For this review, take the finished solid that the model builds, in its own axes (mm). A direction names the side the tool comes from. Round coordinates to 2 decimals unless told otherwise and drop trailing zeros. Order: outer loops, then holes, each group sorted by start corner. A loop starts at its lowest first (then second) coordinate and runs counter-clockwise, first axis right, second up. Notation, with made-up numbers: (10.5, 89.25) -> (60.5, 89.25) arc R17 cw to (60.5, 113.25) -> close; hole circle Ø3 at (18.25, 17.5). An arc over 180 degrees is marked (long way). Answer in a Markdown table with one row per item.
```python
from build123d import *
from build123d.topology import SkipClean

# Parameters (mm, degrees)
SKETCH1_R           = 4
SKETCH1_R_2         = 13
BOSS_EXTRUDE1_DEPTH = 3
BOSS_EXTRUDE2_START = 5
SKETCH2_R           = 17
SKETCH2_R_2         = 8
BOSS_EXTRUDE2_DEPTH = 5
SKETCH3_R           = 1.55
SKETCH3_R_2         = 1
CUT_EXTRUDE1_DEPTH  = 8
SKETCH4_R           = 3.5
SKETCH4_R_2         = 2.2
CUT_EXTRUDE2_DEPTH  = 4.5
SKETCH5_W           = 50
SKETCH5_H           = 15
SKETCH5_R           = 1.55
BOSS_EXTRUDE3_DEPTH = 5
SKETCH9_W           = 42.373333334
SKETCH9_H           = 64.15
BOSS_EXTRUDE6_DEPTH = 3
SKETCH11_R          = 1.55
SKETCH11_R_2        = 4.5
BOSS_EXTRUDE7_DEPTH = 5
SKETCH12_R          = 1.55
BOSS_EXTRUDE8_DEPTH = 4
SKETCH13_R          = 3.5
CUT_EXTRUDE3_DEPTH  = 3


with BuildPart() as part:
    # Sketch1 → Boss-Extrude1 (new body)
    with BuildSketch(Plane.XY):
        with BuildLine():
            Line((-25, 0), (25, 0))
            Line((25, 0), (17, 150))
            ThreePointArc((17, 150), (0, 167), (-17, 150))
            Line((-17, 150), (-25, 0))
        make_face()
        with Locations((0, 150)):
            Circle(SKETCH1_R, mode=Mode.SUBTRACT)
        with Locations((0, 90)):
            Circle(SKETCH1_R_2, mode=Mode.SUBTRACT)
    extrude(amount=BOSS_EXTRUDE1_DEPTH)

    # Sketch2 → Boss-Extrude2 (add)
    with SkipClean():  # the faces are left unmerged after this step: merging them gives an invalid solid
        with BuildSketch(Plane(origin=(0, 0, 0), x_dir=(-1, 0, 0), z_dir=(0, 0, -1)).offset(BOSS_EXTRUDE2_START)):
            with Locations((0, 150)):
                Circle(SKETCH2_R)
            with Locations((0, 150)):
                Circle(SKETCH2_R_2, mode=Mode.SUBTRACT)
        extrude(amount=-BOSS_EXTRUDE2_DEPTH)

    # Sketch3 → Cut-Extrude1 (cut)
    with SkipClean():  # the faces are left unmerged after this step: merging them gives an invalid solid
        with BuildSketch(Plane.XY.offset(3)):
            with Locations((-12.5, 150)):
                Circle(SKETCH3_R)
            with Locations((0, 162.5)):
                Circle(SKETCH3_R)
            with Locations((12.5, 150)):
                Circle(SKETCH3_R)
            with Locations((0, 137.5)):
                Circle(SKETCH3_R)
            with Locations((8.980256121, 158.980256121)):
                Circle(SKETCH3_R_2)
            with Locations((8.980256121, 141.019743879)):
                Circle(SKETCH3_R_2)
            with Locations((-8.980256121, 141.019743879)):
                Circle(SKETCH3_R_2)
            with Locations((-8.980256121, 158.980256121)):
                Circle(SKETCH3_R_2)
        extrude(amount=-CUT_EXTRUDE1_DEPTH, mode=Mode.SUBTRACT)

    # Sketch4 → Cut-Extrude2 (cut)
    with SkipClean():  # the faces are left unmerged after this step: merging them gives an invalid solid
        with BuildSketch(Plane.XY.offset(3)):
            with Locations((-12.5, 150)):
                Circle(SKETCH4_R)
            with Locations((0, 162.5)):
                Circle(SKETCH4_R)
            with Locations((12.5, 150)):
                Circle(SKETCH4_R)
            with Locations((0, 137.5)):
                Circle(SKETCH4_R)
            with Locations((-8.980256121, 158.980256121)):
                Circle(SKETCH4_R_2)
            with Locations((8.980256121, 158.980256121)):
                Circle(SKETCH4_R_2)
            with Locations((8.980256121, 141.019743879)):
                Circle(SKETCH4_R_2)
            with Locations((-8.980256121, 141.019743879)):
                Circle(SKETCH4_R_2)
        extrude(amount=-CUT_EXTRUDE2_DEPTH, mode=Mode.SUBTRACT)

    # Sketch5 → Boss-Extrude3 (add)
    with SkipClean():  # the faces are left unmerged after this step: merging them gives an invalid solid
        with BuildSketch(Plane.XZ):
            with Locations((0, 1.5)):
                Rectangle(SKETCH5_W, SKETCH5_H)
            with Locations((-12.5, 6)):
                Circle(SKETCH5_R, mode=Mode.SUBTRACT)
            with Locations((0, 6)):
                Circle(SKETCH5_R, mode=Mode.SUBTRACT)
            with Locations((12.5, 6)):
                Circle(SKETCH5_R, mode=Mode.SUBTRACT)
            with Locations((0, -3)):
                Circle(SKETCH5_R, mode=Mode.SUBTRACT)
            with Locations((-12.5, -3)):
                Circle(SKETCH5_R, mode=Mode.SUBTRACT)
            with Locations((12.5, -3)):
                Circle(SKETCH5_R, mode=Mode.SUBTRACT)
        extrude(amount=-BOSS_EXTRUDE3_DEPTH)

    # Sketch9 → Boss-Extrude6 (add)
    with SkipClean():  # the faces are left unmerged after this step: merging them gives an invalid solid
        with BuildSketch(Plane.XZ.offset(-71.5)):
            with Locations((0, 35.075)):
                Rectangle(SKETCH9_W, SKETCH9_H)
        extrude(amount=BOSS_EXTRUDE6_DEPTH)

    # Sketch11 → Boss-Extrude7 (add)
    with SkipClean():  # the faces are left unmerged after this step: merging them gives an invalid solid
        with BuildSketch(Plane.XY.offset(51.65)):
            with BuildLine():
                Line((-13, 90), (-13, 71.5))
                Line((-13, 71.5), (13, 71.5))
                Line((13, 71.5), (13, 90))
                ThreePointArc((13, 90), (0, 103), (-13, 90))
            make_face()
            with Locations((-8.5, 90)):
                Circle(SKETCH11_R, mode=Mode.SUBTRACT)
            with Locations((8.5, 90)):
                Circle(SKETCH11_R, mode=Mode.SUBTRACT)
            with Locations((0, 90)):
                Circle(SKETCH11_R_2, mode=Mode.SUBTRACT)
        extrude(amount=BOSS_EXTRUDE7_DEPTH)

    # Sketch12 → Boss-Extrude8 (add)
    # profile 1 of 2: a face of its own
    with SkipClean():  # the faces are left unmerged after this step: merging them gives an invalid solid
        with BuildSketch(Plane.XY.offset(67.15)):
            with BuildLine():
                Line((-11.686666667, 61.5), (-11.686666667, 68.5))
                Line((-11.686666667, 68.5), (-2.686666667, 68.5))
                Line((-2.686666667, 68.5), (-2.686666667, 61.5))
                ThreePointArc((-2.686666667, 61.5), (-7.186666667, 57), (-11.686666667, 61.5))
            make_face()
            with Locations((-7.186666667, 61.5)):
                Circle(SKETCH12_R, mode=Mode.SUBTRACT)
        # profile 2 of 2: a face of its own
        with BuildSketch(Plane.XY.offset(67.15)):
            with BuildLine():
                Line((2.686666667, 61.5), (2.686666667, 68.5))
                Line((2.686666667, 68.5), (11.686666667, 68.5))
                Line((11.686666667, 68.5), (11.686666667, 61.5))
                ThreePointArc((11.686666667, 61.5), (7.186666667, 57), (2.686666667, 61.5))
            make_face()
            with Locations((7.186666667, 61.5)):
                Circle(SKETCH12_R, mode=Mode.SUBTRACT)
        extrude(amount=-BOSS_EXTRUDE8_DEPTH)

    # Sketch13 → Cut-Extrude3 (cut)
    with SkipClean():  # the faces are left unmerged after this step: merging them gives an invalid solid
        with BuildSketch(Plane.XY.offset(56.65)):
            with Locations((-8.5, 90)):
                Circle(SKETCH13_R)
            with Locations((8.5, 90)):
                Circle(SKETCH13_R)
        extrude(amount=-CUT_EXTRUDE3_DEPTH, mode=Mode.SUBTRACT)


solid = part.part
```
Q1. Clearance check with flat-ended pins moving along their axes: pin 1 Ø5.5 at (y, z) = (80, 53.5) entering from +X; pin 2 Ø4.5 at (x, y) = (9, 62.5) entering from -Z; pin 3 Ø8 at (x, y) = (-1.5, 100.5) entering from +Z. State where each tip first meets the part, or that it passes through.
Answer key:
| item | result |
|---|---|
| pin 1 | stops at x = 13 |
| pin 2 | stops at z = 0 |
| pin 3 | stops at z = 56.65 |
Q2. Take a section at A-A, the plane y = 24. Write out the cut boundary in (x, z), then the cut area to 3 significant figures.
Answer key:
| item | result |
|---|---|
| outline | (-23.72, 0) -> (23.72, 0) -> (23.72, 3) -> (-23.72, 3) -> close |
| area | 142 mm^2 |
Q3. The part is to be moulded in two halves that separate along Z. For faces 1 (the face through (-8, 142, -1.5)), 2 (the face through (-13.64, 2.46, 7.05)), 3 (the face through (-12.836, 148.487, -3.226)), say which applies: +Z half, -Z half, draft (parallel to the pull), parting line (faces both ways), or undercut.
Answer key:
| item | result |
|---|---|
| face 1 | +Z half |
| face 2 | undercut |
| face 3 | draft |
Q4. Tool access review of faces 4 (the face through (7.3, 57, 65.2)), 5 (the face through (-8, 88, 53.65)), 6 (the face through (0, 103, 54)), 7 (the face through (11.36, 2.46, 7.05)), 8 (the face through (-11.687, 65, 65)): name each direction out of +Z, -Z, +X, -X, +Y, -Y from which nothing blocks a thin tool from reaching the whole face with its end or side.
Answer key:
| item | result |
|---|---|
| face 4 | +Z, -Y |
| face 5 | +Z |
| face 6 | +Z, +Y |
| face 7 | -Y |
| face 8 | +Z, -X, -Y |
Q5. Take a section at B-B, the plane z = 46.5. Write out the cut boundary in (x, y).
Answer key:
| item | result |
|---|---|
| outline | (-21.19, 68.5) -> (21.19, 68.5) -> (21.19, 71.5) -> (-21.19, 71.5) -> close |
Q6. To check wall thickness, follow probe 1 along Z at (x, y) = (-12.5, 1.6); probe 2 along Y at (x, z) = (0, 10); probe 3 along Z at (x, y) = (-13, 33.5). State the ranges of each line that lie inside material, in increasing order.
Answer key:
| item | result |
|---|---|
| probe 1 | z = -6 to -4.55, -1.45 to 4.45, 7.55 to 9 |
| probe 2 | y = 68.5 to 71.5 |
| probe 3 | z = 0 to 3 |
